from build123d import *

# Parameters (mm, degrees)
BOSS_EXTRUDE1_DEPTH = 23.876
SHELL1_T            = -0.254
SKETCH2_R           = 7.239
CUT_EXTRUDE1_DEPTH  = 0.254
CHAMFER1_SIZE       = 0.254
SKETCH3_R           = 1.524
CUT_EXTRUDE2_DEPTH  = 0.127
SKETCH9_R           = 4.572
CUT_EXTRUDE3_DEPTH  = 0.254
SKETCH18_W          = 2.286
SKETCH18_H          = 0.254
BOSS_EXTRUDE5_DEPTH = 1.651
CUT_EXTRUDE4_DEPTH  = 3.302
SKETCH20_W          = 3.302
SKETCH20_H          = 0.254
BOSS_EXTRUDE6_DEPTH = 0.254
CUT_EXTRUDE5_DEPTH  = 2.667
BOSS_EXTRUDE7_DEPTH = 0.254


with BuildPart() as part:
    # Sketch1 → Boss-Extrude1 (new body)
    with BuildSketch(Plane.XY):
        Polygon((0, 0), (40.64, 0), (12.7, 28.956), (0, 28.956), align=None)
    extrude(amount=-BOSS_EXTRUDE1_DEPTH)

    # Shell1
    shell1_openings = [part.faces().sort_by_distance(p)[0] for p in [
        (20.32, 0, -11.938),
    ]]
    offset(amount=SHELL1_T, openings=shell1_openings, kind=Kind.INTERSECTION)

    # Sketch2 → Cut-Extrude1 (cut)
    with BuildSketch(Plane.ZY):
        with Locations((-11.938, 14.859)):
            Circle(SKETCH2_R)
    extrude(amount=-CUT_EXTRUDE1_DEPTH, mode=Mode.SUBTRACT)

    # Chamfer1
    chamfer1_edges = [part.edges().sort_by_distance(p)[0] for p in [
        (0, 14.859, -19.177),
    ]]
    chamfer(chamfer1_edges, length=CHAMFER1_SIZE - 0.0001)  # a hair under: the kernel refuses the full size

    # Sketch3 → Cut-Extrude2 (cut)
    with BuildSketch(Plane(origin=(21.045482945, 20.307044947, 0), x_dir=(0, 0, -1), z_dir=(0.7196189619724784, 0.6943691738330935, 0))):
        with Locations(Location((19.812, 4.144798155, 0), (0, 0, 90))):
            Circle(SKETCH3_R)
        with Locations(Location((19.812, -20.345163225, 0), (0, 0, 90))):
            Circle(SKETCH3_R)
        with Locations(Location((4.064, 4.144798155, 0), (0, 0, 90))):
            Circle(SKETCH3_R)
        with Locations(Location((4.064, -20.345163225, 0), (0, 0, 90))):
            Circle(SKETCH3_R)
    extrude(amount=-CUT_EXTRUDE2_DEPTH, mode=Mode.SUBTRACT)

    # Sketch9 → Cut-Extrude3 (cut)
    with BuildSketch(Plane(origin=(0, 28.956, 0), x_dir=(1, 0, 0), z_dir=(0, 1, 0))):
        with Locations((9.652, 11.938)):
            Circle(SKETCH9_R)
    extrude(amount=-CUT_EXTRUDE3_DEPTH, mode=Mode.SUBTRACT)

    # Sketch18 → Boss-Extrude5 (add, symmetric)
    with BuildSketch(Plane.XY.offset(-11.938)):
        with Locations((11.557, 28.829)):
            Rectangle(SKETCH18_W, SKETCH18_H)
    extrude(amount=BOSS_EXTRUDE5_DEPTH, both=True)

    # Sketch19 → Cut-Extrude4 (cut)
    with BuildSketch(Plane(origin=(0, 28.956, 0), x_dir=(1, 0, 0), z_dir=(0, 1, 0))):
        with BuildLine():
            Line((10.414, 10.287), (12.065, 10.287))
            ThreePointArc((12.065, 10.287), (10.897566704, 10.770566704), (10.414, 11.938))
            Line((10.414, 11.938), (10.414, 10.287))
        make_face()
        with BuildLine():
            Line((10.414, 13.589), (10.414, 11.938))
            ThreePointArc((10.414, 11.938), (10.897566704, 13.105433296), (12.065, 13.589))
            Line((12.065, 13.589), (10.414, 13.589))
        make_face()
    extrude(amount=-CUT_EXTRUDE4_DEPTH, mode=Mode.SUBTRACT)

    # Sketch20 → Boss-Extrude6 (add)
    with BuildSketch(Plane(origin=(12.7, 0, 0), x_dir=(0, 0, -1), z_dir=(1, 0, 0))):
        with Locations((11.938, 28.829)):
            Rectangle(SKETCH20_W, SKETCH20_H)
    extrude(amount=BOSS_EXTRUDE6_DEPTH)

    # Sketch22 → Cut-Extrude5 (cut, symmetric)
    with BuildSketch(Plane.XY.offset(-11.938)):
        Polygon((12.7, 28.956), (12.954, 28.702), (12.954, 28.956), align=None)
    extrude(amount=CUT_EXTRUDE5_DEPTH, both=True, mode=Mode.SUBTRACT)

    # Sketch23 → Boss-Extrude7 (add)
    with BuildSketch(Plane.XZ):
        with BuildLine():
            Line((39.652035426, -13.589), (40.287035426, -13.589))
            Line((40.287035426, -13.589), (40.287035426, -10.287))
            Line((40.287035426, -10.287), (39.652035426, -10.287))
            ThreePointArc((39.652035426, -10.287), (38.001035426, -11.938), (39.652035426, -13.589))
        make_face()
    extrude(amount=-BOSS_EXTRUDE7_DEPTH)


solid = part.part
Read the model definition and answer for the solid it produces. Units are mm, in the model's axes. A direction names the side the tool comes from. Coordinates: 2 decimals unless noted, no trailing zeros. Order: outer loops, then holes, each group sorted by start corner. A loop starts at its lowest first (then second) coordinate and runs counter-clockwise, first axis right, second up. Notation, with made-up numbers: (49.25, 20) - (93.25, 20) arc R29 ccw to (93.25, 41) - close; hole circle Ø7 at (49, 10.25). An arc over 180 degrees is marked (long way). Use one line per item in the form item = value.
(1) Straight lines are drawn through the part: L1, parallel to Z at x = 6, y = 4.75; L2, parallel to Y at x = 8.5, z = -7; L3, parallel to X at y = 11.25, z = -22.25. For each, find the intervals that lie inside material, in ascending order.
Computed values:
L1 = -23.88 to -23.62, -0.25 to 0
L2 = 28.7 to 28.96
L3 = 0 to 0.25, 29.43 to 29.78
(2) Given pin 1 Ø5 at (y, z) = (25.5, -19) entering from +X; pin 2 Ø12 at (y, z) = (25, -16) entering from -X; pin 3 Ø1 at (x, z) = (27.5, -21.5) entering from +Y; pin 4 Ø10 at (x, z) = (30.5, -17.5) entering from -Y, each flat-ended and moving along its own axis, determine where each tip first touches the part or whether it passes through.
Computed values:
pin_1 = 18.35
pin_2 = 0
pin_3 = 14.14
pin_4 = 4.96
(3) Section C-C, the plane z = -14.5 is taken. Give the number of separate pieces and of enclosed holes in the cut face, then the cut area to 3 significant figures.
Computed values:
separate_pieces = 3
enclosed_holes = 0
area = 15.4 mm²
(4) Which of the six approach directions +Z, -Z, +X, -X, +Y, -Y give full straight-line access (tool end or side, diameter ignored) to faces 1 (the face through (4, 28.956, -12)), 2 (the face through (16, 11, -23.622))?
Computed values:
face_1 = +Z, -Z, +X, -X, +Y
face_2 = -Y
(5) Section D-D, the plane x = 25 is taken. Give the vertices of the cut face in (y, z), then the cut area to 3 significant figures.
Computed values:
outline = (0, -23.88) - (16.21, -23.88) - (16.21, 0) - (0, 0) - (0, -0.25) - (15.84, -0.25) - (15.84, -23.62) - (0, -23.62) - close
area = 16.8 mm²
(6) Section B-B, the plane y = 2.25 is taken. Give the vertices of the cut face in (x, z).
Computed values:
outline = (0, -23.88) - (38.47, -23.88) - (38.47, 0) - (0, 0) - close; hole (0.25, -23.62) - (38.12, -23.62) - (38.12, -0.25) - (0.25, -0.25) - close
(7) Section A-A, the plane x = 9 is taken. Give the vertices of the cut face in (y, z).
Computed values:
outline = (0, -23.88) - (28.96, -23.88) - (28.96, -16.46) - (28.7, -16.46) - (28.7, -23.62) - (0, -23.62) - close; (0, -0.25) - (28.7, -0.25) - (28.7, -7.41) - (28.96, -7.41) - (28.96, 0) - (0, 0) - close
